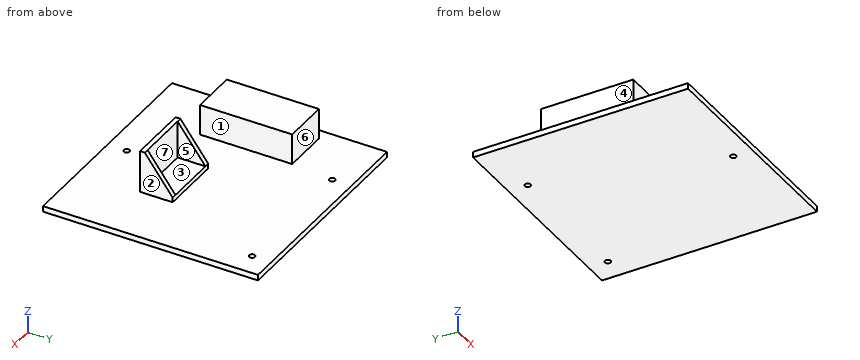
from build123d import *

# Parameters (mm, degrees)
SKETCH1_W           = 116
SKETCH1_H           = 112
BOSS_EXTRUDE1_DEPTH = 3
SKETCH2_W           = 24
SKETCH2_H           = 48
BOSS_EXTRUDE2_DEPTH = 16
SKETCH3_W           = 32
SKETCH3_H           = 17
BOSS_EXTRUDE3_DEPTH = 22
CUT_EXTRUDE1_REACH  = 86
SKETCH5_W           = 27
SKETCH5_H           = 14.5
CUT_EXTRUDE2_DEPTH  = 19.5
CUT_EXTRUDE3_REACH  = 5
SKETCH6_R           = 1.5


with BuildPart() as part:
    # Sketch1 → Boss-Extrude1 (new body)
    with BuildSketch(Plane.XY):
        Rectangle(SKETCH1_W, SKETCH1_H)
    extrude(amount=BOSS_EXTRUDE1_DEPTH)

    # Sketch2 → Boss-Extrude2 (add)
    with BuildSketch(Plane.XY.offset(3)):
        with Locations((-40, 0)):
            Rectangle(SKETCH2_W, SKETCH2_H)
    extrude(amount=BOSS_EXTRUDE2_DEPTH)

    # Sketch3 → Boss-Extrude3 (add)
    with BuildSketch(Plane.XY.offset(3)):
        with Locations((10, -15.5)):
            Rectangle(SKETCH3_W, SKETCH3_H)
    extrude(amount=BOSS_EXTRUDE3_DEPTH)

    # Sketch4 → Cut-Extrude1 (cut, up to next)
    with BuildSketch(Plane(origin=(26, 0, 0), x_dir=(0, 0, -1), z_dir=(1, 0, 0)), mode=Mode.PRIVATE) as cut_extrude1_sk1:
        Polygon((-25, -21.5), (-5.5, -7), (-25, -7), align=None)
    cut_extrude1_tool1 = extrude(cut_extrude1_sk1.sketch, amount=-CUT_EXTRUDE1_REACH, mode=Mode.PRIVATE) & part.part
    add(cut_extrude1_tool1.solids().sort_by_distance((26, -11.833333, 18.5))[0], mode=Mode.SUBTRACT)

    # Sketch5 → Cut-Extrude2 (cut)
    with BuildSketch(Plane.XY.offset(25)):
        with Locations((10, -14.25)):
            Rectangle(SKETCH5_W, SKETCH5_H)
    extrude(amount=-CUT_EXTRUDE2_DEPTH, mode=Mode.SUBTRACT)

    # Sketch6 → Cut-Extrude3 (cut, up to next)
    with BuildSketch(Plane.XY.offset(3), mode=Mode.PRIVATE) as cut_extrude3_sk1:
        with Locations((-26, 46)):
            Circle(SKETCH6_R)
    cut_extrude3_tool1 = extrude(cut_extrude3_sk1.sketch, amount=-CUT_EXTRUDE3_REACH, mode=Mode.PRIVATE) & part.part
    add(cut_extrude3_tool1.solids().sort_by_distance((-26, 46, 3))[0], mode=Mode.SUBTRACT)
    # Sketch6 → Cut-Extrude3 (cut, up to next)
    with BuildSketch(Plane.XY.offset(3), mode=Mode.PRIVATE) as cut_extrude3_sk2:
        with Locations((46, 46)):
            Circle(SKETCH6_R)
    cut_extrude3_tool2 = extrude(cut_extrude3_sk2.sketch, amount=-CUT_EXTRUDE3_REACH, mode=Mode.PRIVATE) & part.part
    add(cut_extrude3_tool2.solids().sort_by_distance((46, 46, 3))[0], mode=Mode.SUBTRACT)
    # Sketch6 → Cut-Extrude3 (cut, up to next)
    with BuildSketch(Plane.XY.offset(3), mode=Mode.PRIVATE) as cut_extrude3_sk3:
        with Locations((0, -46)):
            Circle(SKETCH6_R)
    cut_extrude3_tool3 = extrude(cut_extrude3_sk3.sketch, amount=-CUT_EXTRUDE3_REACH, mode=Mode.PRIVATE) & part.part
    add(cut_extrude3_tool3.solids().sort_by_distance((0, -46, 3))[0], mode=Mode.SUBTRACT)


solid = part.part
For this review, take the finished solid that the model builds, in its own axes (mm). Face numbers are marked on the shaded views. A direction names the side the tool comes from. Give positions to 0.01 mm unless a question says otherwise; leave off trailing zeros. Loops run counter-clockwise (first coordinate to the right, second up) from the corner with the lowest first, then second, coordinate; pieces in that order, holes last.
Item 1: Take a section at A-A, the plane x = 46. State the section outline as (y, z) points.
Item 2: Take a section at B-B, the plane y = 46. State the section outline as (x, z) points.
Item 3: Draft analysis for pull direction X (two halves, no side actions). For the marked faces 4, 5, 6 and 7, state which applies: +X half, -X half, draft (parallel to the pull), parting line (faces both ways), or undercut.
Item 4: Tool access review of the marked faces 1, 2 and 3: name each direction out of +Z, -Z, +X, -X, +Y, -Y from which nothing blocks a thin tool from reaching the whole face with its end or side.
Item 5: For line 1 along Y through (x, z) = (-26, 1.45); line 2 along Y through (x, z) = (-43.5, 8.25); line 3 along Z through (x, y) = (-9, -28), list the stretches that pass through material, from the lowest coordinate up.
Item 6: Insertion check: pin 1 (10 mm diameter, centred on x = -31.5, z = 13, fed in from +Y); pin 2 (5 mm diameter, centred on y = 7, z = 9, fed in from +X); pin 3 (2 mm diameter, centred on x = 29, y = -7.5, fed in from +Z). Each pin has a flat end and moves straight along its axis. Give the tip position at first contact, or say it passes through.
Item 7: Take a section at D-D, the plane y = 8. State the section outline as (x, z) points.
Item 8: Take a section at C-C, the plane z = 13. State the section outline as (x, y) points, and give its area (3 significant figures).
Calculated:
1. outline: (-56, 0) - (44.5, 0) - (44.5, 3) - (-56, 3) - close; (47.5, 0) - (56, 0) - (56, 3) - (47.5, 3) - close
2. outline: (-58, 0) - (-27.5, 0) - (-27.5, 3) - (-58, 3) - close; (-24.5, 0) - (44.5, 0) - (44.5, 3) - (-24.5, 3) - close; (47.5, 0) - (58, 0) - (58, 3) - (47.5, 3) - close
3. face 4: -X half
3. face 5: undercut
3. face 6: draft
3. face 7: undercut
4. face 1: +Z, +Y, -Y
4. face 2: +Z, +X, +Y, -Y
4. face 3: +Z, +Y
5. line 1: y = -56 to 44.5, 47.5 to 56
5. line 2: y = -24 to 24
5. line 3: z = 0 to 3
6. pin 1: stops at y = 24
6. pin 2: stops at x = -28
6. pin 3: stops at z = 3
7. outline: (-58, 0) - (58, 0) - (58, 3) - (-28, 3) - (-28, 19) - (-52, 19) - (-52, 3) - (-58, 3) - close
8. outline: (-52, -24) - (-28, -24) - (-28, 24) - (-52, 24) - close; (-6, -24) - (26, -24) - (26, -12.58) - (23.5, -12.58) - (23.5, -21.5) - (-3.5, -21.5) - (-3.5, -12.58) - (-6, -12.58) - close
8. area: 1,280 mm2
